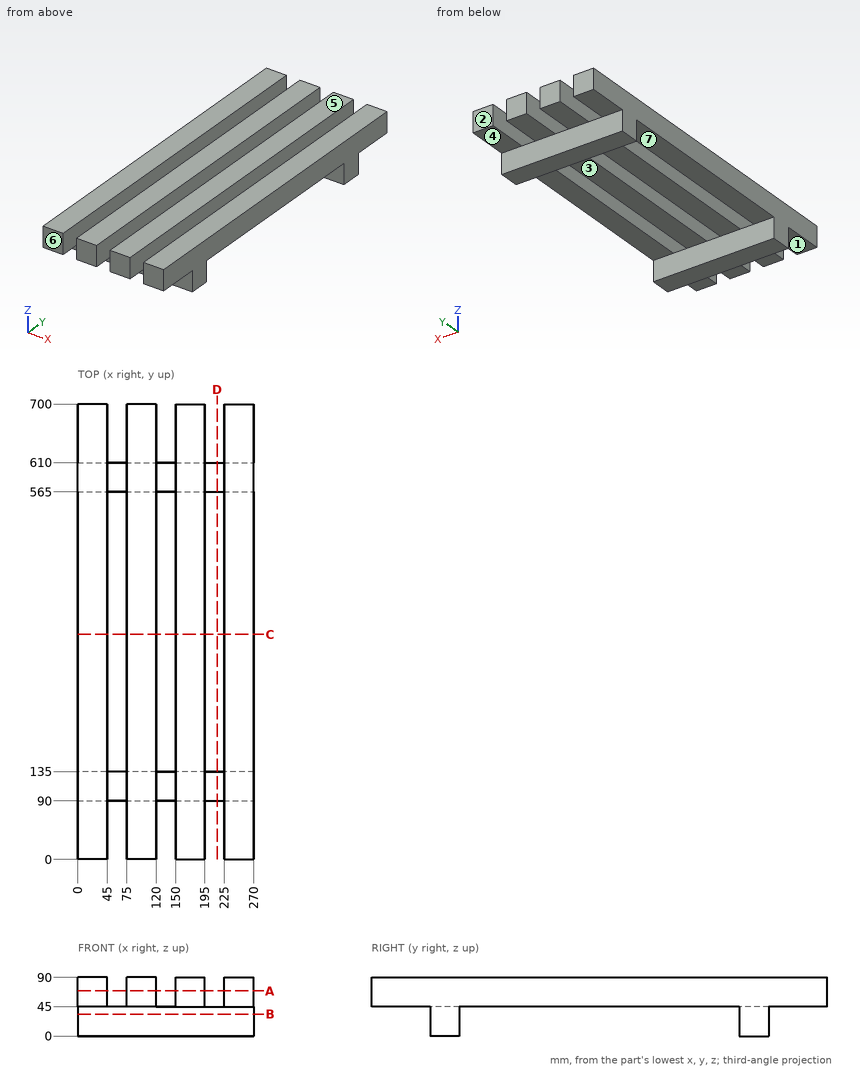
Source: three-view drawing plus pictorial views. Frame: mm from the lowest corner of the part. A direction names the side the tool comes from. Coordinates: 2 decimals unless noted, no trailing zeros. Write each loop counter-clockwise with the first axis right and the second up, starting at its lowest first coordinate (ties: lowest second). Pieces come first, ordered by that corner, then holes. Notation, with made-up numbers: (-29.5, 23.25) -> (3.5, 23.25) arc R18 ccw to (3.5, 37.25) -> close; hole circle Ø5 at (-35.75, -9). An arc over 180 degrees is marked (long way). Write each question's results on one line, items separated by ' | '.
Item 1: Set-up query: the marked faces 1, 2, 3 and 4. Return all of +Z, -Z, +X, -X, +Y, -Y with unobstructed straight access to the full face (end or side cutting, diameter ignored); none if empty.
Conclusion:
face 1: -Z, +X, -X, -Y | face 2: +Z, -Z, +X, -X, +Y | face 3: -Z, +X, -X | face 4: -Z, +X, -X, +Y
Item 2: Section query C-C on y = 346. Return loops of the section in (x, z), plus the area to 3 significant figures.
Conclusion:
outline: (0, 45) -> (45, 45) -> (45, 90) -> (0, 90) -> close; (75, 45) -> (120, 45) -> (120, 90) -> (75, 90) -> close; (150, 45) -> (195, 45) -> (195, 90) -> (150, 90) -> close; (225, 45) -> (270, 45) -> (270, 90) -> (225, 90) -> close | area: 8,100 mm^2
Item 3: Mould query, pull axis Y, two halves, no side actions, for the marked faces 5, 6 and 7. Classes: +Y half, -Y half, draft (parallel to the pull), parting line (faces both ways), or undercut.
Conclusion:
face 5: draft | face 6: -Y half | face 7: undercut
Item 4: Material intervals for probe 1 along X at (y, z) = (598.5, 55); probe 2 along Y at (x, z) = (198.5, 25); probe 3 along Z at (x, y) = (154.5, 213), sorted ascending.
Conclusion:
probe 1: x = 0 to 45, 75 to 120, 150 to 195, 225 to 270 | probe 2: y = 90 to 135, 565 to 610 | probe 3: z = 45 to 90
Item 5: Section query A-A on z = 69.5. Return loops of the section in (x, y).
Conclusion:
outline: (0, 0) -> (45, 0) -> (45, 700) -> (0, 700) -> close; (75, 0) -> (120, 0) -> (120, 700) -> (75, 700) -> close; (150, 0) -> (195, 0) -> (195, 700) -> (150, 700) -> close; (225, 0) -> (270, 0) -> (270, 700) -> (225, 700) -> close
Item 6: Pin query (flat end, axial travel): pin 1 Ø3 at (x, y) = (32, 507) entering from -Z; pin 2 Ø22.5 at (x, z) = (89.5, 12.5) entering from +Y; pin 3 Ø5 at (x, z) = (54.5, 15.5) entering from -Y. Return the tip coordinate at first contact, or that it passes through.
Conclusion:
pin 1: stops at z = 45 | pin 2: stops at y = 610 | pin 3: stops at y = 90
Item 7: Section query B-B on z = 33.5. Return loops of the section in (x, y).
Conclusion:
outline: (0, 90) -> (270, 90) -> (270, 135) -> (0, 135) -> close; (0, 565) -> (270, 565) -> (270, 610) -> (0, 610) -> close
Item 8: Section query D-D on x = 214. Return loops of the section in (y, z), plus the area to 3 significant figures.
Conclusion:
outline: (90, 0) -> (135, 0) -> (135, 45) -> (90, 45) -> close; (565, 0) -> (610, 0) -> (610, 45) -> (565, 45) -> close | area: 4,050 mm^2
